Check sheet for the drawn part. Datum: minimum x, y, z corner. Units: mm. Round coordinates to 2 decimals unless told otherwise and drop trailing zeros. Loops run counter-clockwise (first coordinate to the right, second up) from the corner with the lowest first, then second, coordinate; pieces in that order, holes last.
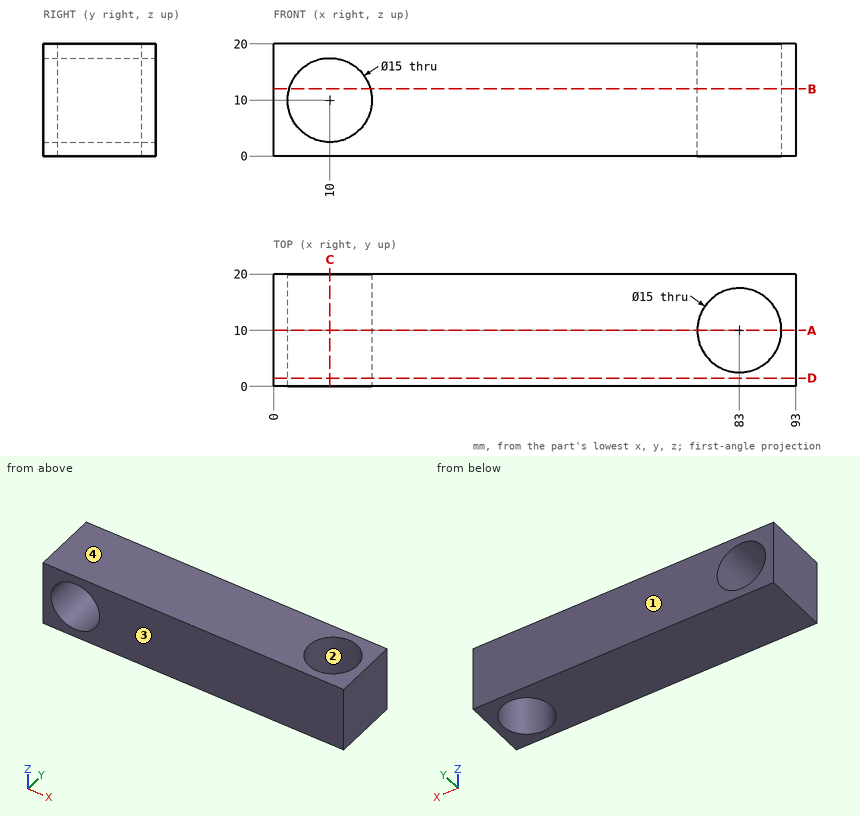
1. Release check for a two-part mould opening along Y. For the marked faces 1, 2, 3 and 4 record: released by +Y, released by -Y, zero draft, split by the parting line, or undercut.
2. Section check B-B (z = 12). Enter the section's corners in (x, y).
3. Section check D-D (y = 1.5). Enter the section's corners in (x, z).
4. Section check A-A (y = 10). Enter the section's corners in (x, z).
5. Scan lines: L1, parallel to Z at x = 10, y = 7.25; L2, parallel to X at y = 4.5, z = 6.75. Record each from-to range of solid material in increasing order.
6. Section check C-C (x = 10). Enter the section's corners in (y, z), then the cut area to 3 significant figures.
7. Gauge pin test, flat ends, axial feed: P1, Ø3, axis at y = 8.5, z = 9.5, coming from the -X side; P2, Ø2, axis at x = 9.5, z = 15, coming from the -Y side. Record the tip position at first contact, or that the pin passes through.
Taken from the geometry:
1. face 1: released by +Y
1. face 2: undercut
1. face 3: released by -Y
1. face 4: zero draft
2. outline: (0, 0) - (2.77, 0) - (2.77, 20) - (0, 20) - close; (17.23, 0) - (93, 0) - (93, 20) - (17.23, 20) - close; hole circle Ø15 at (83, 10)
3. outline: (0, 0) - (93, 0) - (93, 20) - (0, 20) - close; hole circle Ø15 at (10, 10)
4. outline: (0, 0) - (75.5, 0) - (75.5, 20) - (0, 20) - close; (90.5, 0) - (93, 0) - (93, 20) - (90.5, 20) - close; hole circle Ø15 at (10, 10)
5. L1: z = 0 to 2.5, 17.5 to 20
5. L2: x = 0 to 3.24, 16.76 to 77.9, 88.1 to 93
6. outline: (0, 0) - (20, 0) - (20, 2.5) - (0, 2.5) - close; (0, 17.5) - (20, 17.5) - (20, 20) - (0, 20) - close
6. area: 100 mm2
7. P1: stops at x = 0
7. P2: passes through
